Design review of the part built by this model. Coordinates are the model's own, in mm. A direction names the side the tool comes from. Give positions to 0.01 mm unless a question says otherwise; leave off trailing zeros. Loops run counter-clockwise (first coordinate to the right, second up) from the corner with the lowest first, then second, coordinate; pieces in that order, holes last. Notation, with made-up numbers: (75.25, 7) - (89.25, 7) arc R22 cw to (89.25, 29) - close; hole circle Ø6 at (86, -18). An arc over 180 degrees is marked (long way). Write each question's results on one line, items separated by ' | '.
from build123d import *

# Parameters (mm, degrees)
SKETCH1_R           = 95.25
SKETCH1_R_2         = 88.9
BOSS_EXTRUDE1_DEPTH = 50.8
BOSS_EXTRUDE2_START = -0.850464
SKETCH2_R           = 12.7
BOSS_EXTRUDE2_DEPTH = 26.250464
SKETCH3_R           = 3.175
CUT_EXTRUDE1_DEPTH  = 50.8
FILLET1_R           = 1.27
SKETCH4_R           = 3.175
CUT_EXTRUDE2_DEPTH  = 10.16


with BuildPart() as part:
    # Sketch1 → Boss-Extrude1 (new body)
    with BuildSketch(Plane(origin=(0, 0, 0), x_dir=(1, 0, 0), z_dir=(0, 1, 0))):
        with Locations(Location((0, 0, 0), (0, 0, 270))):
            Circle(SKETCH1_R)
        with Locations(Location((0, 0, 0), (0, 0, 270))):
            Circle(SKETCH1_R_2, mode=Mode.SUBTRACT)
    extrude(amount=BOSS_EXTRUDE1_DEPTH)

    # Sketch2 → Boss-Extrude2 (add)
    with BuildSketch(Plane.ZY.offset(95.25).offset(BOSS_EXTRUDE2_START)):
        with Locations(Location((0, 25.4, 0), (0, 0, 180))):
            Circle(SKETCH2_R)
    boss_extrude2 = extrude(amount=BOSS_EXTRUDE2_DEPTH)

    # Sketch3 → Cut-Extrude1 (cut)
    with BuildSketch(Plane.ZY.offset(120.65)):
        with Locations((0, 25.4)):
            Circle(SKETCH3_R)
    cut_extrude1 = extrude(amount=-CUT_EXTRUDE1_DEPTH, mode=Mode.SUBTRACT)

    # Mirror1: Boss-Extrude2, Cut-Extrude1 across plane
    add(boss_extrude2.mirror(Plane(origin=(0, 0, 0), x_dir=(0, 0, 1), z_dir=(1, 0, 0))))
    add(cut_extrude1.mirror(Plane(origin=(0, 0, 0), x_dir=(0, 0, 1), z_dir=(1, 0, 0))), mode=Mode.SUBTRACT)

    # Fillet1
    fillet1_edges = [part.edges().sort_by_distance(p)[0] for p in [
        (-120.65, 25.4, 12.7),
        (-120.65, 25.4, -3.175),
        (120.65, 25.4, 12.7),
        (120.65, 25.4, -3.175),
    ]]
    fillet(fillet1_edges, radius=FILLET1_R)

    # Sketch4 → Cut-Extrude2 (cut)
    with BuildSketch(Plane(origin=(0, 0, -95.25), x_dir=(-1, 0, 0), z_dir=(0, 0, -1))):
        with Locations(Location((0, 25.4, 0), (0, 0, 90))):
            Circle(SKETCH4_R)
    cut_extrude2 = extrude(amount=-CUT_EXTRUDE2_DEPTH, mode=Mode.SUBTRACT)

    # Mirror2: Cut-Extrude2 across plane
    add(cut_extrude2.mirror(Plane.XY), mode=Mode.SUBTRACT)


solid = part.part
(1) Take a section at B-B on x = 0. Give the boundary of the cut face in (y, z) (3 decimals), plus the area to 3 significant figures.
Answers below:
outline: (0, -95.25) - (22.225, -95.25) - (22.225, -88.9) - (0, -88.9) - close; (0, 88.9) - (22.225, 88.9) - (22.225, 95.25) - (0, 95.25) - close; (28.575, -95.25) - (50.8, -95.25) - (50.8, -88.9) - (28.575, -88.9) - close; (28.575, 88.9) - (50.8, 88.9) - (50.8, 95.25) - (28.575, 95.25) - close | area: 565 mm2
(2) Take a section at D-D on x = -38. Give the boundary of the cut face in (y, z), plus the area to 3 significant figures.
Answers below:
outline: (0, -87.34) - (50.8, -87.34) - (50.8, -80.37) - (0, -80.37) - close; (0, 80.37) - (50.8, 80.37) - (50.8, 87.34) - (0, 87.34) - close | area: 708 mm2
(3) Insertion check: P1, Ø5, axis at y = 35, z = -23, coming from the +X side; P2, Ø6, axis at x = 55, y = 20, coming from the +Z side; P3, Ø3, axis at x = 38.5, y = 20, coming from the -Z side. Each pin has a flat end and moves straight along its axis. Give the tip position at first contact, or say it passes through.
Answers below:
P1: x = 93.02 | P2: z = 79.8 | P3: z = -87.77
(4) Tool access review of faces 5 (the cylindrical face through (-106.71, 37.8, 2.75)), 6 (the flat face through (43, 50.8, -78)): name each direction out of +Z, -Z, +X, -X, +Y, -Y from which nothing blocks a thin tool from reaching the whole face with its end or side.
Answers below:
face 5: -X | face 6: +Z, -Z, +X, -X, +Y
(5) Draft analysis for pull direction Y (two halves, no side actions). For faces 1 (the cylindrical face through (-1.22, 28.33, 92.09)), 2 (the cylindrical face through (106.71, 37.8, 2.75)), 3 (the cylindrical face through (104.33, 28.55, -0.41)), 4 (the flat face through (43, 0, -78)), state which applies: pulls with the +Y half, pulls with the -Y half, needs draft (parallel to the pull), parting line crosses it, or undercut.
Answers below:
face 1: undercut | face 2: parting line crosses it | face 3: undercut | face 4: pulls with the -Y half
(6) Take a section at A-A on z = 0. Count the separate pieces of the cut face and the enclosed holes in it, plus the area to 3 significant figures.
Answers below:
separate pieces: 4 | enclosed holes: 0 | area: 1,530 mm2
(7) Wall thickness on line 1 along Z through (x, y) = (110.5, 25.4) (3 decimals); line 2 along Z through (x, y) = (1.5, 47.5); line 3 along Y through (x, z) = (-109.5, 0) (3 decimals): over which ranges is each line inside the solid? List them lowest first. Write a range as from..to.
Answers below:
line 1: -12.7..-3.175, 3.175..12.7 | line 2: -95.24..-88.89, 88.89..95.24 | line 3: 12.7..22.225, 28.575..38.1
